Read the model definition and answer for the solid it produces. Units are mm, in the model's axes. Face numbers are marked on the shaded views. A direction names the side the tool comes from. Round coordinates to 2 decimals unless told otherwise and drop trailing zeros. Loops run counter-clockwise (first coordinate to the right, second up) from the corner with the lowest first, then second, coordinate; pieces in that order, holes last. Notation, with made-up numbers: M 14,66 L 69,66 A10 ccw 69,85 Z; hole C 45.5,11.25 d8. An arc over 180 degrees is marked long. Answer as CSV lines item,"result".
```python
from build123d import *

# Parameters (mm, degrees)
F0_R     = 9.9949
F0_R_2   = 5.7023
F1_DEPTH = 19.5072
F0_R_3   = 29.9974
F0_R_4   = 8.001
F2_DEPTH = 13.462
F0_R_5   = 35.0012
F3_DEPTH = 15.0114


with BuildPart() as f1:
    # F0 (on Front) → F1 (new body)
    with BuildSketch(Plane.XZ):
        Circle(F0_R)
        Circle(F0_R_2, mode=Mode.SUBTRACT)
    extrude(amount=F1_DEPTH)

    # F0 (on Front) → F2 (join)
    with BuildSketch(Plane.XZ):
        Circle(F0_R_3)
        with Locations((-0.396391, -21.008808)):
            Circle(F0_R_4, mode=Mode.SUBTRACT)
        with Locations((21.008808, -0.396391)):
            Circle(F0_R_4, mode=Mode.SUBTRACT)
        with Locations((-21.008808, 0.396391)):
            Circle(F0_R_4, mode=Mode.SUBTRACT)
        Circle(F0_R, mode=Mode.SUBTRACT)
        with Locations((0.396391, 21.008808)):
            Circle(F0_R_4, mode=Mode.SUBTRACT)
    extrude(amount=F2_DEPTH)

    # F0 (on Front) → F3 (join)
    with BuildSketch(Plane.XZ):
        Circle(F0_R_5)
        Circle(F0_R_3, mode=Mode.SUBTRACT)
    extrude(amount=F3_DEPTH)


solid = f1.part
```
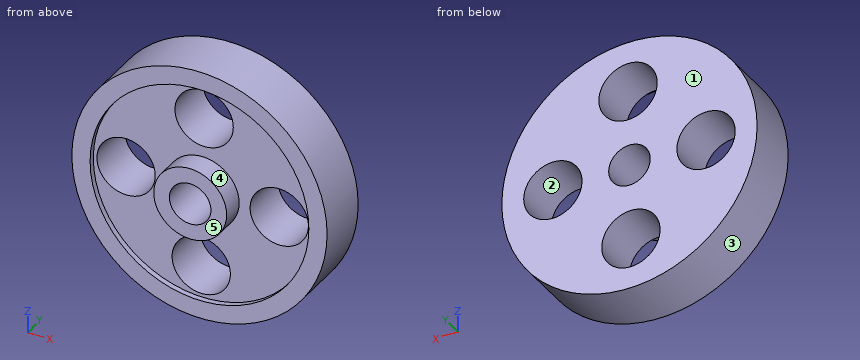
1) A tool of negligible diameter and unlimited length cuts with its end or side. For the marked faces 4 and 5, from which of +Z, -Z, +X, -X, +Y, -Y can it reach the whole face along a straight path? Write none if from no direction.
Evaluation:
face 4,"-Y"
face 5,"+Z, -Z, +X, -X, -Y"
2) Each of these flat-tipped pins is pushed along its axis until it touches: P1, Ø1.5, axis at x = 6.5, y = -17, coming from the +Z side; P2, Ø3, axis at x = 7, y = -4, coming from the -Z side; P3, Ø14.5, axis at x = -21.01, z = 0.4, coming from the -Y side; P4, Ø1, axis at x = 15.5, y = -9, coming from the +Z side. Where does it stop, or does it pass through?
Evaluation:
P1,"stops at z = 8.18"
P2,"stops at z = -34.57"
P3,"passes through"
P4,"stops at z = 31.62"
3) Straight lines are drawn through the part: line 1 (Z direction, x = 0, y = -7); line 2 (Z direction, x = 0, y = -13.75); line 3 (X direction, y = -13.25, z = 2). For each, find the intervals that lie inside material, in ascending order.
Evaluation:
line 1,"z = -35 to -29, -13.02 to -5.7, 5.7 to 13.02, 29 to 35"
line 2,"z = -35 to -30, -9.99 to -5.7, 5.7 to 9.99, 30 to 35"
line 3,"x = -34.94 to -28.85, -13.17 to -5.34, 5.34 to 13.38, 28.64 to 34.94"
4) Find section C-C, the plane z = 2. Give the vertices of the cut face in (x, y).
Evaluation:
outline,"M -34.94,-15.01 L -29.93,-15.01 L -29.93,-13.46 L -28.85,-13.46 L -28.85,0 L -34.94,0 Z; M -13.17,-13.46 L -9.79,-13.46 L -9.79,-19.51 L -5.34,-19.51 L -5.34,0 L -13.17,0 Z; M 5.34,-19.51 L 9.79,-19.51 L 9.79,-13.46 L 13.38,-13.46 L 13.38,0 L 5.34,0 Z; M 28.64,-13.46 L 29.93,-13.46 L 29.93,-15.01 L 34.94,-15.01 L 34.94,0 L 28.64,0 Z"
5) Find section D-D, the plane y = -2.5. Give the vertices of the cut face in (x, z).
Evaluation:
outline,"C 0,0 d70; hole C -21.01,0.4 d16; hole C -0.4,-21.01 d16; hole C 0.4,21.01 d16; hole C 0,0 d11.4; hole C 21.01,-0.4 d16"
6) Find section A-A, the plane x = 0. Give the vertices of the cut face in (y, z).
Evaluation:
outline,"M -19.51,-9.99 L -13.46,-9.99 L -13.46,-13.02 L 0,-13.02 L 0,-5.7 L -19.51,-5.7 Z; M -19.51,5.7 L 0,5.7 L 0,13.02 L -13.46,13.02 L -13.46,9.99 L -19.51,9.99 Z; M -15.01,-35 L 0,-35 L 0,-29 L -13.46,-29 L -13.46,-30 L -15.01,-30 Z; M -15.01,30 L -13.46,30 L -13.46,29 L 0,29 L 0,35 L -15.01,35 Z"
7) Find section B-B, the plane z = -24. Give the vertices of the cut face in (x, y), then the cut area to 3 significant figures.
Evaluation:
outline,"M -25.48,-15.01 L -18,-15.01 L -18,-13.46 L -7.82,-13.46 L -7.82,0 L -25.48,0 Z; M 7.02,-13.46 L 18,-13.46 L 18,-15.01 L 25.48,-15.01 L 25.48,0 L 7.02,0 Z"
area,"509 mm^2"
8) Determine the mould class of the marked faces 1, 2 and 3 for opening direction X: released by +X, released by -X, zero draft, split by the parting line, or undercut.
Evaluation:
face 1,"zero draft"
face 2,"undercut"
face 3,"split by the parting line"
